Check sheet for the modelled part. Datum: model origin and axes. Units: mm. A direction names the side the tool comes from. Coordinates: 2 decimals unless noted, no trailing zeros. Order: outer loops, then holes, each group sorted by start corner. A loop starts at its lowest first (then second) coordinate and runs counter-clockwise, first axis right, second up.
1. Draft check along Z on faces 1 (the cylindrical face through (9.08, 1.01, 13.52)), 2 (the flat face through (7, 1, 0)), 3 (the cylindrical face through (4.51, 20.53, 2.31)). Enter one of: released by +Z, released by -Z, zero draft, split by the parting line, or undercut.
2. Cross-section at D-D (z = 17). Enter the section's corners in (x, y), then the cut area to 3 significant figures.
3. Cross-section at C-C (x = 10.75). Enter the section's corners in (y, z).
4. Thickness scan on line 1 (Z direction, x = 6.75, y = 15.5); line 2 (Y direction, x = 7.75, z = 7.75); line 3 (Y direction, x = 0.5, z = 8.5). Record the ranges inside material, lowest first.
5. Cross-section at A-A (z = 12.5). Enter the section's corners in (x, y), then the cut area to 3 significant figures.
6. Set-up check for faces 4 (the flat face through (11, 20, 1.82)), 5 (the flat face through (13.001, 20, 3)), 6 (the flat face through (6.61, 22.45, 2.82)), 7 (the flat face through (8.13, 2, 10.55)): record each of +Z, -Z, +X, -X, +Y, -Y from which the full face is reachable in a straight line by a thin tool's end or side.
7. Cross-section at B-B (y = 19). Enter the section's corners in (x, z), then the cut area to 3 significant figures.
8. Gauge pin test, flat ends, axial feed: pin 1 Ø1.5 at (x, z) = (6.5, 22) entering from +Y; pin 2 Ø5 at (x, y) = (7.26, 20.5) entering from -Z; pin 3 Ø5.5 at (x, y) = (9.5, 13.5) entering from -Z. Record the tip position at first contact, or that the pin passes through.
```python
from build123d import *

# Parameters (mm, degrees)
SKETCH_1_W          = 15
SKETCH_1_H          = 25
EXTRUDE_1_DEPTH     = 3
CUT_EXTRUDE_1_DEPTH = 1
SKETCH_3_R          = 1.9
CUT_EXTRUDE_2_DEPTH = 30.223278392
SKETCH_4_W          = 11.000545076
SKETCH_4_H          = 1.5
EXTRUDE_2_DEPTH     = 35
CUT_EXTRUDE_3_DEPTH = 1
SKETCH_6_R          = 1.9
CUT_EXTRUDE_4_DEPTH = 10


with BuildPart() as part:
    # 草图1 → 凸台-拉伸1 (new body)
    with BuildSketch(Plane(origin=(0, 0, 0), x_dir=(1, 0, 0), z_dir=(0, 1, 0))):
        with Locations((7.5, -12.5)):
            Rectangle(SKETCH_1_W, SKETCH_1_H)
    extrude(amount=EXTRUDE_1_DEPTH)

    # 草图2 → 切除-拉伸1 (cut)
    with BuildSketch(Plane(origin=(0, 3, 0), x_dir=(1, 0, 0), z_dir=(0, 1, 0))):
        with BuildLine():
            Line((9.229285522, -6), (9.229285522, -10.378679656))
            ThreePointArc((9.229285522, -10.378679656), (10.229285522, -12.5), (9.229285522, -14.621320344))
            Line((9.229285522, -14.621320344), (9.229285522, -19))
            ThreePointArc((9.229285522, -19), (7.479285522, -20.75), (5.729285522, -19))
            Line((5.729285522, -19), (5.729285522, -14.621320344))
            ThreePointArc((5.729285522, -14.621320344), (4.729285522, -12.5), (5.729285522, -10.378679656))
            Line((5.729285522, -10.378679656), (5.729285522, -6))
            ThreePointArc((5.729285522, -6), (7.479285522, -4.25), (9.229285522, -6))
        make_face()
    extrude(amount=-CUT_EXTRUDE_1_DEPTH, mode=Mode.SUBTRACT)

    # 草图3 → 切除-拉伸2 (cut, through all)
    with BuildSketch(Plane(origin=(0, 2, 0), x_dir=(1, 0, 0), z_dir=(0, 1, 0))):
        with Locations(Location((7.479285522, -12.5, 0), (0, 0, 270))):
            Circle(SKETCH_3_R)
    extrude(amount=-CUT_EXTRUDE_2_DEPTH, mode=Mode.SUBTRACT)

    # 草图4 → 凸台-拉伸2 (add)
    with BuildSketch(Plane(origin=(0, 3, 0), x_dir=(1, 0, 0), z_dir=(0, 1, 0))):
        with Locations((7.500272538, -2.569906393)):
            Rectangle(SKETCH_4_W, SKETCH_4_H)
    extrude(amount=EXTRUDE_2_DEPTH)

    # 草图5 → 切除-拉伸3 (cut)
    with BuildSketch(Plane(origin=(0, 0, 1.819906393), x_dir=(-1, 0, 0), z_dir=(0, 0, -1))):
        with BuildLine():
            Line((-9.008775904, 14), (-9.008775904, 18.378679656))
            ThreePointArc((-9.008775904, 18.378679656), (-10.008775904, 20.5), (-9.008775904, 22.621320344))
            Line((-9.008775904, 22.621320344), (-9.008775904, 27))
            ThreePointArc((-9.008775904, 27), (-7.258775904, 28.75), (-5.508775904, 27))
            Line((-5.508775904, 27), (-5.508775904, 22.621320344))
            ThreePointArc((-5.508775904, 22.621320344), (-4.508775904, 20.5), (-5.508775904, 18.378679656))
            Line((-5.508775904, 18.378679656), (-5.508775904, 14))
            ThreePointArc((-5.508775904, 14), (-7.258775904, 12.25), (-9.008775904, 14))
        make_face()
    extrude(amount=-CUT_EXTRUDE_3_DEPTH, mode=Mode.SUBTRACT)

    # 草图6 → 切除-拉伸4 (cut)
    with BuildSketch(Plane(origin=(0, 0, 2.819906393), x_dir=(-1, 0, 0), z_dir=(0, 0, -1))):
        with Locations((-7.258775904, 20.5)):
            Circle(SKETCH_6_R)
    extrude(amount=-CUT_EXTRUDE_4_DEPTH, mode=Mode.SUBTRACT)


solid = part.part
```
Data:
1. face 1: undercut
1. face 2: released by -Z
1. face 3: zero draft
2. outline: (0, 0) - (15, 0) - (15, 3) - (9.23, 3) - (9.23, 2) - (5.73, 2) - (5.73, 3) - (0, 3) - close
2. area: 41.5 mm2
3. outline: (0, 0) - (3, 0) - (3, 1.82) - (38, 1.82) - (38, 3.32) - (3, 3.32) - (3, 25) - (0, 25) - close
4. line 1: z = 2.82 to 3.32
4. line 2: y = 0 to 2
4. line 3: y = 0 to 3
5. outline: (0, 0) - (5.58, 0) - (5.58, 2) - (4.73, 2) - (4.73, 3) - (0, 3) - close; (9.38, 0) - (15, 0) - (15, 3) - (10.23, 3) - (10.23, 2) - (9.38, 2) - close
5. area: 31.9 mm2
6. face 4: -Z, +X, -X, +Y
6. face 5: +Z, -Z, +X, +Y
6. face 6: -Z
6. face 7: +Y
7. outline: (2, 1.82) - (4.95, 1.82) - (4.95, 2.82) - (6.09, 2.82) - (6.09, 3.32) - (2, 3.32) - close; (8.42, 2.82) - (9.56, 2.82) - (9.56, 1.82) - (13, 1.82) - (13, 3.32) - (8.42, 3.32) - close
7. area: 10.7 mm2
8. pin 1: stops at y = 3
8. pin 2: stops at z = 2.82
8. pin 3: stops at z = 1.82
